The listing builds one solid part. Answer for the finished solid, in the listing's coordinates (mm). A direction names the side the tool comes from. Coordinates: 2 decimals unless noted, no trailing zeros. Write each loop counter-clockwise with the first axis right and the second up, starting at its lowest first coordinate (ties: lowest second). Pieces come first, ordered by that corner, then holes.
(1) Which of the six approach directions +Z, -Z, +X, -X, +Y, -Y give full straight-line access (tool end or side, diameter ignored) to faces 4 (the flat face through (-10.615, -18.427, 24.65)), 5 (the flat face through (-34.2, -23.2, 24.7)), 6 (the flat face through (65.76, 26.42, 23.42))?
(2) The part is cut by section D-D on y = -10.5. Determine the outline of the cut face in (x, z), plus the area to 3 significant figures.
(3) Given P1, Ø6, axis at x = -54.5, z = 42, coming from the -Y side; P2, Ø1, axis at y = -5.5, z = 5.5, coming from the +X side; P3, Ø1, axis at x = -50, y = -32, coming from the -Z side; P4, Ø11.5, axis at x = 46.58, y = 23.72, coming from the -Z side, each flat-ended and moving along its own axis, determine where each tip first touches the part or whether it passes through.
(4) The part is cut by section B-B on x = -45.5. Determine the outline of the cut face in (y, z), plus the area to 3 significant figures.
(5) The part is cut by section C-C on z = 4. Give the number of separate pieces and of enclosed holes in the cut face, plus the area to 3 significant figures.
(6) For a pull along X with two mould halves and no side action, classify faces 1 (the flat face through (19, 2, 50)), 2 (the flat face through (1, 46.524, 23)), 3 (the flat face through (67.66, 28.04, 24.65)) as +X half, -X half, draft (parallel to the pull), parting line (faces both ways), or undercut.
(7) The part is cut by section A-A on y = -36.5. Determine the outline of the cut face in (x, z), plus the area to 3 significant figures.
(8) Straight lines are drawn through the part: line 1 (Y direction, x = -43, z = 8.5); line 2 (X direction, y = -37.5, z = 20.5); line 3 (X direction, y = -33, z = 10.5). For each, find the intervals that lie inside material, in ascending order.
from build123d import *

# Parameters (mm, degrees)
F0_R     = 6.35
F1_DEPTH = 50
F2_R     = 4
F3_T     = -2.5
F5_D     = 6.7564
F6_SIZE  = 5


with BuildPart() as f1:
    # F0 (on Top) → F1 (new body)
    with BuildSketch(Plane.XY):
        Polygon((49.709592275, 49.0236406618), (-49.350407725, 49.0236406618), (-51.6386922998, 44.4470657872), (-29.6711277494, 13.3263486253), (-88.8431668297, -48.1600951648), (-34.8197797575, -42.9655389343), (-36.9358653545, -20.9582477999), (13.6309133433, -16.0960577452), (32.8233957422, -42.9655389343), (83.6233957422, -42.9655389343), (84.9492279691, 7.8344567721), align=None)
        with Locations((46.5822630314, 23.7201556859)):
            Circle(F0_R, mode=Mode.SUBTRACT)
    extrude(amount=F1_DEPTH)

    # F2
    f2_edges = [f1.edges().sort_by_distance(p)[0] for p in [
        (84.949228, 7.834457, 25),
        (83.623396, -42.965539, 25),
        (-34.81978, -42.965539, 25),
        (32.823396, -42.965539, 25),
        (-88.843167, -48.160095, 25),
        (49.709592, 49.023641, 25),
        (-29.671128, 13.326349, 25),
        (-51.638692, 44.447066, 25),
        (13.630913, -16.096058, 25),
    ]]
    fillet(f2_edges, radius=F2_R)

    # F3
    f3_openings = [f1.faces().sort_by_distance(p)[0] for p in [
        (13.724729, 2.432943, 0),
    ]]
    offset(amount=F3_T, openings=f3_openings, kind=Kind.INTERSECTION)

    # F5 (through all)
    with Locations(Plane.XY.offset(50)):
        with Locations((-6.9581352872, 13.156432332), (-16.0837286401, 28.0593003633)):
            Hole(F5_D / 2)

    # F6
    f6_edges = [f1.edges().sort_by_distance(p)[0] for p in [
        (-36.935865, -20.958248, 25),
    ]]
    chamfer(f6_edges, length=F6_SIZE)


solid = f1.part
Model answer:
1. face 4: +Z, -Z, -Y
1. face 5: +Z, -Z
1. face 6: -Z
2. outline: (-52.6, 0) - (-49.13, 0) - (-49.13, 47.5) - (81.97, 47.5) - (81.97, 0) - (84.47, 0) - (84.47, 50) - (-52.6, 50) - close
2. area: 626 mm2
3. P1: stops at y = -45.15
3. P2: stops at x = 84.61
3. P3: stops at z = 47.5
3. P4: passes through
4. outline: (-43.99, 0) - (-41.48, 0) - (-41.48, 47.5) - (-6.73, 47.5) - (-6.73, 0) - (-3.12, 0) - (-3.12, 50) - (-43.99, 50) - close; (35.75, 0) - (40.09, 0) - (40.09, 47.5) - (46.52, 47.5) - (46.52, 0) - (49.02, 0) - (49.02, 50) - (35.75, 50) - close
4. area: 751 mm2
5. separate pieces: 2
5. enclosed holes: 2
5. area: 1,430 mm2
6. face 1: draft
6. face 2: undercut
6. face 3: +X half
7. outline: (-77.62, 0) - (-74.15, 0) - (-74.15, 47.5) - (-37.95, 47.5) - (-37.95, 0) - (-35.44, 0) - (-35.44, 50) - (-77.62, 50) - close; (28.21, 0) - (31.28, 0) - (31.28, 47.5) - (81.29, 47.5) - (81.29, 0) - (83.79, 0) - (83.79, 50) - (28.21, 50) - close
7. area: 793 mm2
8. line 1: y = -43.75 to -41.24, -4.13 to -0.52, 32.21 to 36.54, 46.52 to 49.02
8. line 2: x = -78.58 to -75.11, -37.86 to -35.35, 28.92 to 31.99, 81.27 to 83.77
8. line 3: x = -74.25 to -70.78, -38.29 to -35.78, 25.71 to 28.78, 81.38 to 83.88
